```python
from build123d import *

# Parameters (mm, degrees)
SKETCH1_W            = 10
SKETCH1_H            = 5
BOSS_EXTRUDE1_DEPTH  = 10
SKETCH2_R            = 5
BOSS_EXTRUDE2_DEPTH  = 10
CUT_EXTRUDE1_REACH   = 17
SKETCH3_R            = 3
CUT_EXTRUDE2_DEPTH   = 16
FILLET1_R            = 1
FILLET1_OF_MIRROR1_R = 1


with BuildPart() as part:
    # Sketch1 → Boss-Extrude1 (new body)
    with BuildSketch(Plane(origin=(0, 0, 0), x_dir=(1, 0, 0), z_dir=(0, 1, 0))):
        with Locations((5, 0)):
            Rectangle(SKETCH1_W, SKETCH1_H)
    boss_extrude1 = extrude(amount=BOSS_EXTRUDE1_DEPTH)

    # Sketch2 → Boss-Extrude2 (add)
    with BuildSketch(Plane(origin=(0, 0, 0), x_dir=(1, 0, 0), z_dir=(0, 1, 0))):
        Circle(SKETCH2_R)
    boss_extrude2 = extrude(amount=BOSS_EXTRUDE2_DEPTH)

    # Sketch3 → Cut-Extrude1 (cut, up to next)
    with BuildSketch(Plane(origin=(0, 0, 0), x_dir=(1, 0, 0), z_dir=(0, 1, 0)), mode=Mode.PRIVATE) as cut_extrude1_sk1:
        with Locations(Location((0, 0, 0), (0, 0, 270))):
            Circle(SKETCH3_R)
    cut_extrude1_tool1 = extrude(cut_extrude1_sk1.sketch, amount=CUT_EXTRUDE1_REACH, mode=Mode.PRIVATE) & part.part
    cut_extrude1 = cut_extrude1_tool1.solids().sort_by_distance((0, 0, 0))[0]
    add(cut_extrude1, mode=Mode.SUBTRACT)

    # Sketch4 → Cut-Extrude2 (cut, symmetric)
    with BuildSketch(Plane.XY):
        with BuildLine():
            Line((0, 8), (-5, 8))
            Line((-5, 8), (-5, 2))
            Line((-5, 2), (0, 2))
            ThreePointArc((0, 2), (3, 5), (0, 8))
        make_face()
    cut_extrude2 = extrude(amount=CUT_EXTRUDE2_DEPTH, both=True, mode=Mode.SUBTRACT)

    # Fillet1
    fillet1_edges = [part.edges().sort_by_distance(p)[0] for p in [
        (4.330127019, 5, 2.5),
        (4.330127019, 5, -2.5),
    ]]
    fillet(fillet1_edges, radius=FILLET1_R)

    # Mirror1: Boss-Extrude1, Boss-Extrude2, Cut-Extrude1, Cut-Extrude2 across plane
    add(boss_extrude1.mirror(Plane(origin=(10, 10, -2.5), x_dir=(0, 0, 1), z_dir=(-1, 0, 0))))
    add(boss_extrude2.mirror(Plane(origin=(10, 10, -2.5), x_dir=(0, 0, 1), z_dir=(-1, 0, 0))))
    add(cut_extrude1.mirror(Plane(origin=(10, 10, -2.5), x_dir=(0, 0, 1), z_dir=(-1, 0, 0))), mode=Mode.SUBTRACT)
    add(cut_extrude2.mirror(Plane(origin=(10, 10, -2.5), x_dir=(0, 0, 1), z_dir=(-1, 0, 0))), mode=Mode.SUBTRACT)

    # Fillet1 of Mirror1
    fillet1_of_mirror1_edges = [part.edges().sort_by_distance(p)[0] for p in [
        (15.669872981, 5, 2.5),
        (15.669872981, 5, -2.5),
    ]]
    fillet(fillet1_of_mirror1_edges, radius=FILLET1_OF_MIRROR1_R)


solid = part.part
```
The model under review builds one solid part; all positions refer to its coordinate system, in mm. A direction names the side the tool comes from. Round coordinates to 2 decimals unless told otherwise and drop trailing zeros. Loops run counter-clockwise (first coordinate to the right, second up) from the corner with the lowest first, then second, coordinate; pieces in that order, holes last. Notation, with made-up numbers: (-37.5, 27) -> (-24.5, 27) arc R12 ccw to (-24.5, 40) -> close; hole circle Ø5 at (-29, -26.75). An arc over 180 degrees is marked (long way). Answer in a Markdown table with one row per item.
1) Wall thickness on line 1 along Y through (x, z) = (-2, -4.5); line 2 along Z through (x, y) = (0, 8.2); line 3 along X through (y, z) = (8.75, 0): over which ranges is each line inside the solid? List them lowest first.
Taken from the geometry:
| item | result |
|---|---|
| line 1 | y = 0 to 2, 8 to 10 |
| line 2 | z = -5 to -3, 3 to 5 |
| line 3 | x = -5 to -3, 3 to 17, 23 to 25 |
2) Consider section A-A, the plane y = 8.5. Write out the cut boundary in (x, z), plus the area to 3 significant figures.
Taken from the geometry:
| item | result |
|---|---|
| outline | (4.06, -2.92) arc R1 cw to (4.87, -2.5) -> (15.13, -2.5) arc R1 cw to (15.94, -2.92) arc R5 ccw (long way) to (15.94, 2.92) arc R1 cw to (15.13, 2.5) -> (4.87, 2.5) arc R1 cw to (4.06, 2.92) arc R5 ccw (long way) to start; hole circle Ø6 at (0, 0); hole circle Ø6 at (20, 0) |
| area | 153 mm² |
3) Tool access review of faces 1 (the flat face through (10, 5, -2.5)), 2 (the cylindrical face through (4.42, 4.93, 2.61)), 3 (the flat face through (24, 2, 0)): name each direction out of +Z, -Z, +X, -X, +Y, -Y from which nothing blocks a thin tool from reaching the whole face with its end or side.
Taken from the geometry:
| item | result |
|---|---|
| face 1 | -Z, +Y, -Y |
| face 2 | +Z, +Y, -Y |
| face 3 | +Z, -Z, +X |
4) Consider section D-D, the plane z = -3.5. Write out the cut boundary in (x, y).
Taken from the geometry:
| item | result |
|---|---|
| outline | (-3.57, 0) -> (3.57, 0) -> (3.57, 10) -> (-3.57, 10) -> (-3.57, 8) -> (0, 8) arc R3 cw to (0, 2) -> (-3.57, 2) -> close; (16.43, 0) -> (23.57, 0) -> (23.57, 2) -> (20, 2) arc R3 cw to (20, 8) -> (23.57, 8) -> (23.57, 10) -> (16.43, 10) -> close |
5) For pin 1 Ø1.5 at (x, z) = (-2, 0) entering from -Y; pin 2 Ø5 at (x, y) = (7.5, 5.5) entering from +Z; pin 3 Ø3 at (x, y) = (7.5, 3.5) entering from -Z; pin 4 Ø2 at (x, y) = (2.5, 6) entering from -Z, all flat-tipped, find the tip position at first contact; note any pin that passes through.
Taken from the geometry:
| item | result |
|---|---|
| pin 1 | passes through |
| pin 2 | stops at z = 2.5 |
| pin 3 | stops at z = -2.5 |
| pin 4 | stops at z = -4.46 |
6) Consider section B-B, the plane z = 1.5. Write out the cut boundary in (x, y), plus the area to 3 significant figures.
Taken from the geometry:
| item | result |
|---|---|
| outline | (-4.77, 0) -> (-2.6, 0) -> (-2.6, 2) -> (-4.77, 2) -> close; (-4.77, 8) -> (-2.6, 8) -> (-2.6, 10) -> (-4.77, 10) -> close; (2.6, 0) -> (17.4, 0) -> (17.4, 3.5) arc R3 cw to (17.4, 6.5) -> (17.4, 10) -> (2.6, 10) -> (2.6, 6.5) arc R3 cw to (2.6, 3.5) -> close; (22.6, 0) -> (24.77, 0) -> (24.77, 2) -> (22.6, 2) -> close; (22.6, 8) -> (24.77, 8) -> (24.77, 10) -> (22.6, 10) -> close |
| area | 164 mm² |
7) Consider section C-C, the plane z = 4.5. Write out the cut boundary in (x, y), plus the area to 3 significant figures.
Taken from the geometry:
| item | result |
|---|---|
| outline | (-2.18, 0) -> (2.18, 0) -> (2.18, 2.94) arc R3 cw to (0, 2) -> (-2.18, 2) -> close; (-2.18, 8) -> (0, 8) arc R3 cw to (2.18, 7.06) -> (2.18, 10) -> (-2.18, 10) -> close; (17.82, 0) -> (22.18, 0) -> (22.18, 2) -> (20, 2) arc R3 cw to (17.82, 2.94) -> close; (17.82, 7.06) arc R3 cw to (20, 8) -> (22.18, 8) -> (22.18, 10) -> (17.82, 10) -> close |
| area | 37.4 mm² |
8) Draft analysis for pull direction Y (two halves, no side actions). For faces 4 (the cylindrical face through (15.58, 4.93, 2.61)), 5 (the cylindrical face through (3, 5, 3)), 6 (the flat face through (10, 0, 0)), state which applies: pulls with the +Y half, pulls with the -Y half, needs draft (parallel to the pull), parting line crosses it, or undercut.
Taken from the geometry:
| item | result |
|---|---|
| face 4 | needs draft |
| face 5 | undercut |
| face 6 | pulls with the -Y half |
